Could you check a few things on this model? Use its own coordinates, in mm. A direction names the side the tool comes from. Round coordinates to 2 decimals unless told otherwise and drop trailing zeros. Loops run counter-clockwise (first coordinate to the right, second up) from the corner with the lowest first, then second, coordinate; pieces in that order, holes last. Notation, with made-up numbers: M 17,70.25 L 49,70.25 A7 ccw 49,76.25 Z; hole C 72.25,-27.5 d5. An arc over 180 degrees is marked long. Answer in a Markdown table with one row per item.
```python
from build123d import *

# Parameters (mm, degrees)
BOSS_EXTRU_1_DEPTH      = 5
BOSS_EXTRU_2_DEPTH      = 1
ESQUISSE3_W             = 5.2
ESQUISSE3_H             = 5.2
ESQUISSE3_W_2           = 5
ESQUISSE3_H_2           = 5
ENL_V_MAT_EXTRU_1_DEPTH = 4.8
CONG_4_R                = 2


with BuildPart() as part:
    # Esquisse1 → Boss.-Extru.1 (new body)
    with BuildSketch(Plane(origin=(0, 0, 0), x_dir=(1, 0, 0), z_dir=(0, 1, 0))):
        Polygon((22, 13), (12.003020456, 23), (-12.003020456, 23), (-22, 13), (-22, -13), (-12.003020456, -23), (12.003020456, -23), (22, -13), (22, -5), (26, -5), (26, 5), (22, 5), align=None)
    extrude(amount=BOSS_EXTRU_1_DEPTH)

    # Esquisse2 → Boss.-Extru.2 (add)
    with BuildSketch(Plane(origin=(0, 5, 0), x_dir=(1, 0, 0), z_dir=(0, 1, 0))):
        Polygon((17.001510228, -18), (17.001510228, 18), (-22, 0), align=None)
        Polygon((-10.06810155, 0), (12.001510228, -10.185580242), (12.001510228, 10.185580242), align=None, mode=Mode.SUBTRACT)
    extrude(amount=BOSS_EXTRU_2_DEPTH)

    # Esquisse3 → Enlèv. mat.-Extru.1 (cut)
    with BuildSketch(Plane.XZ):
        with Locations((-13.4, 14.4)):
            Rectangle(ESQUISSE3_W, ESQUISSE3_H)
        with Locations((-13.4, -14.4)):
            Rectangle(ESQUISSE3_W, ESQUISSE3_H)
        with Locations((13.4, -14.4)):
            Rectangle(ESQUISSE3_W, ESQUISSE3_H)
        with Locations((13.4, 14.4)):
            Rectangle(ESQUISSE3_W, ESQUISSE3_H)
        Rectangle(ESQUISSE3_W_2, ESQUISSE3_H_2)
    extrude(amount=-ENL_V_MAT_EXTRU_1_DEPTH, mode=Mode.SUBTRACT)

    # Congé4
    cong_4_edges = [part.edges().sort_by_distance(p)[0] for p in [
        (-22, 5.5, 0),
        (17.001510228, 5.5, 18),
        (17.001510228, 5.5, -18),
    ]]
    fillet(cong_4_edges, radius=CONG_4_R)


solid = part.part
```
1) Which directions (+Z, -Z, +X, -X, +Y, -Y) give clear straight access to the entire face, cutting with the end or side of a thin tool? Please do faces 1 (the face through (13, 4.8, -14)), 2 (the face through (-2.177, 5.493, 9.149)), 3 (the face through (16.103, 5.507, 16.544)), 4 (the face through (16.103, 5.507, -16.544)).
Computed:
| item | result |
|---|---|
| face 1 | -Y |
| face 2 | +Z, -X, +Y |
| face 3 | +Z, +Y |
| face 4 | -Z, +Y |
2) Will these pins go through, and if not, where does the flat tip stop? P1, Ø1.5, axis at y = 2.5, z = -14, coming from the +X side; P2, Ø2.5, axis at x = -14.5, y = 3, coming from the -Z side; P3, Ø2.5, axis at x = -14, y = 1.5, coming from the -Z side.
Computed:
| item | result |
|---|---|
| P1 | stops at x = 21.75 |
| P2 | stops at z = -21.75 |
| P3 | stops at z = -22.25 |
3) I want a section at A-A, the plane y = 1.5. State how many separate pieces and enclosed holes the cut face has, plus the area to 3 significant figures.
Computed:
| item | result |
|---|---|
| separate pieces | 1 |
| enclosed holes | 5 |
| area | 1,730 mm² |
4) I want a section at D-D, the plane z = -18. Please give me the cut outline in (x, y).
Computed:
| item | result |
|---|---|
| outline | M -17,0 L 17,0 L 17,5 L -17,5 Z |
5) I need wall thicknesses on line 1 (Z direction, x = 11.5, y = 2.5); line 2 (Z direction, x = -1, y = 2); line 3 (X direction, y = 2.75, z = 12). Which ranges of each line are inside material? Lowest first, please.
Computed:
| item | result |
|---|---|
| line 1 | z = -23 to -17, -11.8 to 11.8, 17 to 23 |
| line 2 | z = -23 to -2.5, 2.5 to 23 |
| line 3 | x = -22 to -16, -10.8 to 10.8, 16 to 22 |
6) I want a section at B-B, the plane z = 7. Please give me the cut outline in (x, y), plus the area to 3 significant figures.
Computed:
| item | result |
|---|---|
| outline | M -22,0 L 22,0 L 22,5 L 17,5 L 17,6 L 12,6 L 12,5 L 5.1,5 L 5.1,6 L -6.83,6 L -6.83,5 L -22,5 Z |
| area | 237 mm² |
7) I want a section at C-C, the plane x = -8.5. Please give me the cut outline in (y, z), plus the area to 3 significant figures.
Computed:
| item | result |
|---|---|
| outline | M 0,-23 L 5,-23 L 5,-6.23 L 6,-6.23 L 6,-0.72 L 5,-0.72 L 5,0.72 L 6,0.72 L 6,6.23 L 5,6.23 L 5,23 L 0,23 Z |
| area | 241 mm² |
